from build123d import *

# Parameters (mm, degrees)
CYLINDER_R              = 3
CYLINDER_DEPTH          = 15
CYLINDER_PITCH_ANGLE    = -90
CYLINDER001_R           = 3
CYLINDER001_DEPTH       = 15
CYLINDER001_PITCH_ANGLE = -90
PAD_DEPTH               = 10
SKETCH001_R             = 1.7
POCKET_DEPTH            = 20
CHAMFER_SIZE            = 2
CHAMFER001_SIZE         = 0.7
CHAMFER002_SIZE         = 0.5


with BuildPart() as cilindro:
    # Cylinder → Cylinder (new body)
    with BuildSketch(Plane.XY):
        Circle(CYLINDER_R)
    extrude(amount=CYLINDER_DEPTH)


with BuildPart() as cilindro_1:
    # Cylinder pitch: moved
    add(cilindro.part.rotate(Axis((0, 0, 0), (0, 1, 0)), CYLINDER_PITCH_ANGLE))


with BuildPart() as cilindro_2:
    # Cylinder placement: moved
    add(cilindro_1.part.moved(Location((18, 12.5, 5))))


with BuildPart() as fusion:
    # Cylinder001 → Cylinder001 (new body)
    with BuildSketch(Plane.XY):
        Circle(CYLINDER001_R)
    extrude(amount=CYLINDER001_DEPTH)


with BuildPart() as fusion_1:
    # Cylinder001 pitch: moved
    add(fusion.part.rotate(Axis((0, 0, 0), (0, 1, 0)), CYLINDER001_PITCH_ANGLE))


with BuildPart() as fusion_2:
    # Cylinder001 placement: moved
    add(fusion_1.part.moved(Location((18, -12.5, 5))))

    # Fusion: union Cilindro
    add(cilindro_2.part)


with BuildPart() as chamfer002:
    # Sketch → Pad (new body)
    with BuildSketch(Plane.XY):
        with BuildLine():
            ThreePointArc((-8, -14.316424), (16.4, 0), (-8, 14.316424))
            ThreePointArc((-8, 20.493902), (-11.088739, 17.405163), (-8, 14.316424))
            ThreePointArc((0, 22), (-4.070268, 21.620197), (-8, 20.493902))
            Line((0, 22), (22, 22))
            Line((22, 22), (22, -22))
            Line((0, -22), (22, -22))
            ThreePointArc((-8, -20.493902), (-4.070268, -21.620197), (0, -22))
            ThreePointArc((-8, -14.316424), (-11.08874, -17.405163), (-8, -20.493902))
        make_face()
    extrude(amount=PAD_DEPTH)

    # Sketch001 → Pocket (cut)
    with BuildSketch(Plane.YZ.offset(22)):
        with Locations((-12.5, 5)):
            Circle(SKETCH001_R)
        with Locations((12.5, 5)):
            Circle(SKETCH001_R)
    extrude(amount=-POCKET_DEPTH, mode=Mode.SUBTRACT)

    # Cut: cut Fusion
    add(fusion_2.part, mode=Mode.SUBTRACT)

    # Chamfer
    chamfer_edges = [chamfer002.edges().sort_by_distance(p)[0] for p in [
        (-8, -20.493902, 5),
        (-8, 20.493902, 5),
    ]]
    chamfer(chamfer_edges, length=CHAMFER_SIZE)

    # Chamfer001
    chamfer001_edges = [chamfer002.edges().sort_by_distance(p)[0] for p in [
        (16.4, 0, 10),
        (16.4, 0, 0),
    ]]
    chamfer(chamfer001_edges, length=CHAMFER001_SIZE)

    # Chamfer002
    chamfer002_edges = [chamfer002.edges().sort_by_distance(p)[0] for p in [
        (22, 0, 0),
        (22, 0, 10),
    ]]
    chamfer(chamfer002_edges, length=CHAMFER002_SIZE)


solid = chamfer002.part
Verification items for the finished model (mm, model axes). A direction names the side the tool comes from. Coordinates: 2 decimals unless noted, no trailing zeros. Loops run counter-clockwise (first coordinate to the right, second up) from the corner with the lowest first, then second, coordinate; pieces in that order, holes last. Notation, with made-up numbers: M -9,-14 L 21,-14 A17 cw 21,11 Z; hole C 3,-5 d3. An arc over 180 degrees is marked long. One line per item, written item: value.
1. Gauge pin test, flat ends, axial feed: P1, Ø4.5, axis at y = -12.5, z = 5, coming from the -X side; P2, Ø4, axis at y = 9, z = 5, coming from the -X side. Record the tip position at first contact, or that the pin passes through.
Answers follow:
P1: x = -9.58
P2: x = 12.97
2. Section check B-B on z = 5. Give the number of separate pieces and of enclosed holes in the cut face, plus the area to 3 significant figures.
Answers follow:
separate pieces: 3
enclosed holes: 0
area: 547 mm^2
3. Section check A-A on x = 19.5. Record the cut outline in (y, z), plus the area to 3 significant figures.
Answers follow:
outline: M -22,0 L 22,0 L 22,10 L -22,10 Z; hole C -12.5,5 d3.4; hole C 12.5,5 d3.4
area: 422 mm^2
4. Mould release check, pull along Z, two halves, no side actions. Record for faces 3 (the conical face through (16.5, -0.49, 0.59)), 4 (the cylindrical face through (-10.94, 16.46, 4.93)), 5 (the cylindrical face through (20, -11.7, 3.5)): pulls with the +Z half, pulls with the -Z half, needs draft (parallel to the pull), parting line crosses it, or undercut.
Answers follow:
face 3: pulls with the -Z half
face 4: needs draft
face 5: undercut
5. Material ranges on line 1 along Z through (x, y) = (19, 12.5); line 2 along Y through (x, z) = (10.25, 5); line 3 along Y through (x, z) = (-7, 6), recorded low to high. Write a range as from..to.
Answers follow:
line 1: 0..3.3, 6.7..10
line 2: -22..-15.5, 15.5..22
line 3: -20.83..-14.83, 14.83..20.83
6. Set-up check for faces 1 (the flat face through (18, -14.5, 5)), 2 (the cylindrical face through (20, 13.3, 3.5)): record each of +Z, -Z, +X, -X, +Y, -Y from which the full face is reachable in a straight line by a thin tool's end or side.
Answers follow:
face 1: none
face 2: +X, -X
